The model under review builds one solid part; all positions refer to its coordinate system, in mm. Face numbers are marked on the shaded views. A direction names the side the tool comes from. Round coordinates to 2 decimals unless told otherwise and drop trailing zeros. Loops run counter-clockwise (first coordinate to the right, second up) from the corner with the lowest first, then second, coordinate; pieces in that order, holes last. Notation, with made-up numbers: M 70.25,-25.75 L 110.25,-25.75 A5 ccw 110.25,-16.75 Z; hole C 50,1 d10. An arc over 180 degrees is marked long. Use a Markdown table: item, result. Add a question column.
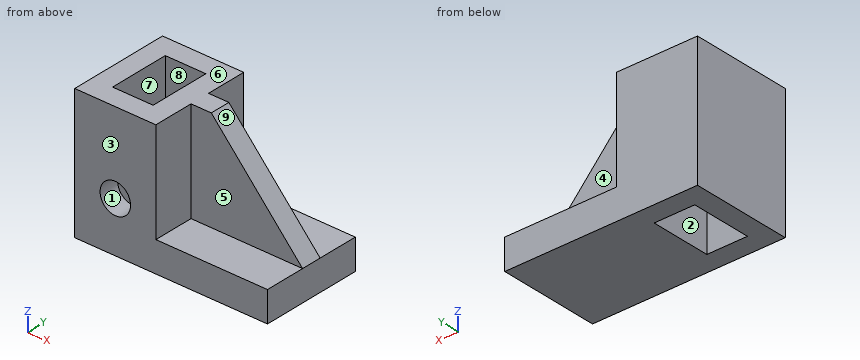
Autodesk Fusion 360 part; units mm, degrees
sketch "Sketch1" plane through (0, 0, 0) normal (0, 1, 0) x (1, 0, 0)
  line L0 (0, 0) -> (95, 0)
  line L1 (95, 0) -> (95, -15)
  line L2 (95, -15) -> (40, -15)
  line L3 (40, -15) -> (40, -65)
  line L4 (40, -65) -> (0, -65)
  line L5 (0, -65) -> (0, 0)
  dimension "d1" = 95
extrude "Extrude1" add sketch "Sketch1" along normal blind 50
sketch "Sketch2" plane through (0, 0, 65) normal (0, 0, 1) x (-1, 0, 0)
  line L0 (0, 0) -> (-40, 0)
  line L1 (-40, 0) -> (-40, -50)
  line L2 (-40, -50) -> (0, -50)
  line L3 (0, -50) -> (0, 0)
  line L4 (7.2091, -40) -> (5, -40)
  line L5 (-10, -10) -> (-30, -10)
  line L6 (-10, -40) -> (-30, -40)
  line L7 (-30, -10) -> (-30, -40)
  line L8 (-10, -10) -> (-10, -40)
extrude "Extrude2" cut sketch "Sketch2" against normal blind 90 contours L5 L6 L7 L8
sketch "Sketch3" plane through (0, 0, 0) normal (0, -1, 0) x (1, 0, 0)
  line L0 (40, 65) -> (0, 65)
  line L1 (0, 65) -> (0, 0)
  line L2 (0, 0) -> (95, 0)
  line L3 (95, 0) -> (95, 15)
  line L4 (95, 15) -> (40, 15)
  line L5 (40, 15) -> (40, 65)
  line L6 (-20, 25) -> (0, 25)
  circle A0 centre (20, 25) radius 7.5
  line L7 (20, 0) -> (20, -6.3794)
  dimension "d15" = 25
  dimension "d16" = 15
extrude "Extrude3" cut sketch "Sketch3" against normal blind 20 contours A0
sketch "Sketch4" plane through (0, 0, 15) normal (0, 0, 1) x (-1, 0, 0)
  line L0 (-40, 0) -> (-95, 0)
  line L1 (-95, 0) -> (-95, -50)
  line L2 (-95, -50) -> (-40, -50)
  line L3 (-40, -50) -> (-40, 0)
  line L4 (-40, -20) -> (-95, -20)
  line L5 (-40, -30) -> (-95, -30)
extrude "Extrude4" add sketch "Sketch4" along normal blind 50 contours L1 L3 L4 L5
sketch "Sketch5" plane through (0, 0, 65) normal (0, 0, 1) x (-1, 0, 0)
  line L0 (-10, -40) -> (-30, -40)
  line L1 (-30, -40) -> (-30, -10)
  line L2 (-30, -10) -> (-10, -10)
  line L3 (-10, -10) -> (-10, -40)
  line L4 (0, 0) -> (-40, 0)
  line L5 (-40, 0) -> (-40, -20)
  line L6 (-40, -30) -> (-40, -50)
  line L7 (-40, -50) -> (0, -50)
  line L8 (0, -50) -> (0, 0)
sketch "Sketch6" plane through (0, 20, 0) normal (0, -1, 0) x (1, 0, 0)
  line L0 (40, 15) -> (95, 15)
  line L1 (95, 15) -> (95, 65)
  line L2 (95, 65) -> (40, 65)
  line L3 (40, 65) -> (40, 15)
  line L4 (50, 65) -> (95, 15)
  point P0 (50, 65)
extrude "Extrude5" cut sketch "Sketch6" against normal blind 65 contours L1 L2 L4
sketch "Sketch7" plane through (0, 0, 0) normal (0, 1, 0) x (1, 0, 0)
(1) Insertion check: pin 1 Ø9 at (y, z) = (19, 37) entering from +X; pin 2 Ø10 at (y, z) = (41.5, 35) entering from +X; pin 3 Ø16 at (x, y) = (70, 8.5) entering from +Z. Each pin has a flat end and moves straight along its axis. Give the tip position at first contact, or say it passes through.
(2) Consider section C-C, the plane y = 3. Give the boundary of the cut face in (x, z), then the cut area to 3 significant figures.
(3) Consider section B-B, the plane z = 12. Give the boundary of the cut face in (x, y).
(4) Consider section A-A, the plane y = 25. Give the boundary of the cut face in (x, z), then the cut area to 3 significant figures.
(5) To check wall thickness, follow probe 1 along Y at (x, z) = (14, 11.5); probe 2 along X at (y, z) = (18, 23.5); probe 3 along Z at (x, y) = (20, 4.75). State the ranges of each line that lie inside material, in increasing order.
(6) Draft analysis for pull direction X (two halves, no side actions). For the marked faces 6, 7, 8 and 9, state which applies: released by +X, released by -X, zero draft, split by the parting line, or undercut.
(7) For the marked faces 1, 2, 3, 4 and 5, list the 3-axis set-ups (+Z, -Z, +X, -X, +Y, -Y) from which the entire face can be reached by the end or side of a thin tool; tool diameter is ignored.
(8) Consider section D-D, the plane x = 20. Give the boundary of the cut face in (y, z).
Found:
| question | item | result |
|---|---|---|
| 1 | pin 1 | stops at x = 79.15 |
| 1 | pin 2 | stops at x = 40 |
| 1 | pin 3 | stops at z = 15 |
| 2 | outline | M 0,0 L 95,0 L 95,15 L 40,15 L 40,65 L 0,65 Z; hole C 20,25 d15 |
| 2 | area | 3,250 mm^2 |
| 3 | outline | M 0,0 L 95,0 L 95,50 L 0,50 Z; hole M 10,10 L 30,10 L 30,40 L 10,40 Z |
| 4 | outline | M 0,0 L 10,0 L 10,65 L 0,65 Z; M 30,0 L 95,0 L 95,15 L 50,65 L 30,65 Z |
| 4 | area | 3,750 mm^2 |
| 5 | probe 1 | y = 0 to 10, 40 to 50 |
| 5 | probe 2 | x = 0 to 10, 30 to 40 |
| 5 | probe 3 | z = 0 to 17.5, 32.5 to 65 |
| 6 | face 6 | zero draft |
| 6 | face 7 | undercut |
| 6 | face 8 | undercut |
| 6 | face 9 | released by +X |
| 7 | face 1 | -Y |
| 7 | face 2 | +Z, -Z |
| 7 | face 3 | +Z, -Z, +X, -X, -Y |
| 7 | face 4 | +Z, +X, +Y |
| 7 | face 5 | +Z, +X, -Y |
| 8 | outline | M 0,0 L 10,0 L 10,17.5 L 0,17.5 Z; M 0,32.5 L 10,32.5 L 10,65 L 0,65 Z; M 40,0 L 50,0 L 50,65 L 40,65 Z |
